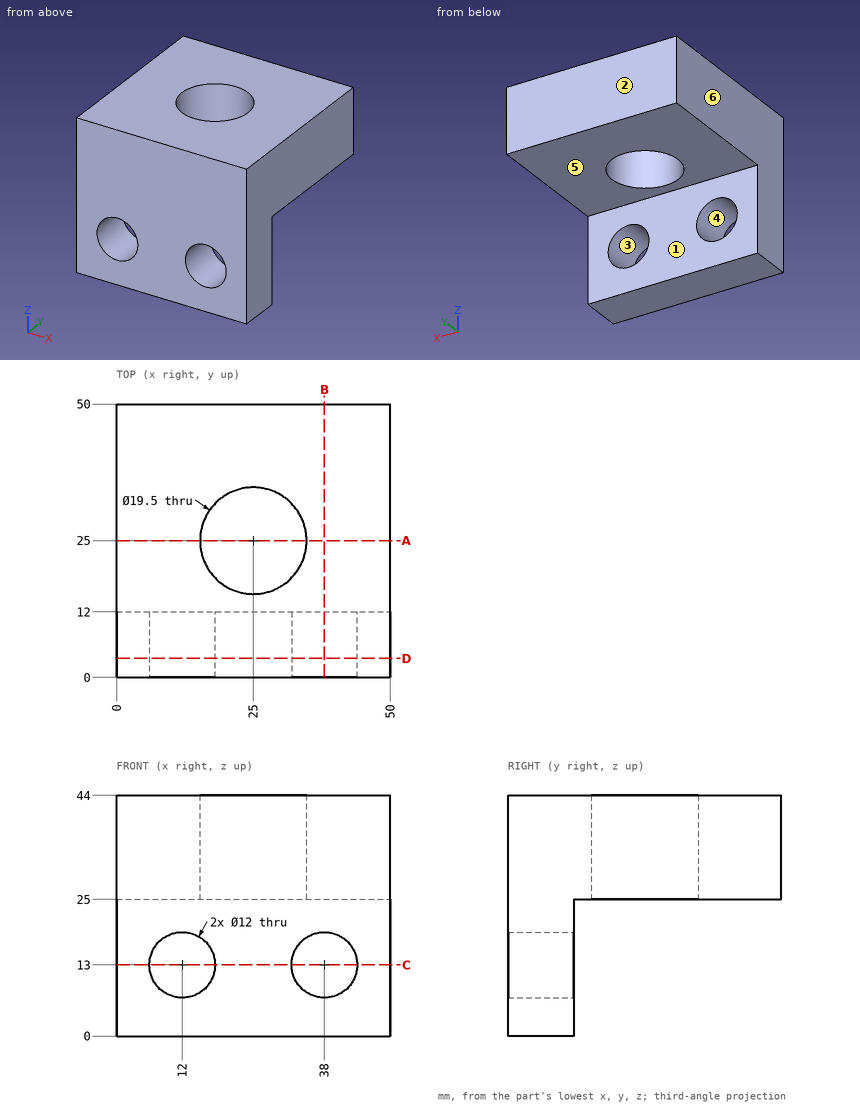
Input: dimensioned drawing with shaded views. Units: mm. Origin: part minimum x, y, z. A direction names the side the tool comes from. Give positions to 0.01 mm unless a question says otherwise; leave off trailing zeros. Write each loop counter-clockwise with the first axis right and the second up, starting at its lowest first coordinate (ties: lowest second). Pieces come first, ordered by that corner, then holes.
1. Material intervals for line 1 along Z through (x, y) = (38, 7); line 2 along Y through (x, z) = (25, 30.5); line 3 along Y through (x, z) = (46.5, 13.5), sorted ascending.
2. First-contact query: pin 1 (3 mm diameter, centred on x = 11, y = 44.5, fed in from -Z); pin 2 (6 mm diameter, centred on x = 30.5, z = 18.5, fed in from +Y). Flat tips, straight axial feed; report the tip coordinate or a pass-through.
3. Pull-direction query (X, two-part tool) for the marked faces 3, 4, 5 and 6; classes: +X half, -X half, draft (parallel to the pull), parting line (faces both ways), or undercut.
4. Access query for the marked faces 1 and 2. Directions: +Z, -Z, +X, -X, +Y, -Y. A direction counts if a zero-diameter tool reaches every point of the face in a straight line with its end or side. Return the directions, or none.
5. Section query D-D (y = 3.5). Return the cut outline in (x, z), then the cut area to 3 significant figures.
6. Section query A-A (y = 25). Return the cut outline in (x, z), then the cut area to 4 significant figures.
7. Section query B-B (x = 38). Return the cut outline in (y, z), then the cut area to 3 significant figures.
8. Section query C-C (z = 13). Return the cut outline in (x, y), then the cut area to 3 significant figures.
Output values:
1. line 1: z = 0 to 7, 19 to 44
1. line 2: y = 0 to 15.25, 34.75 to 50
1. line 3: y = 0 to 12
2. pin 1: stops at z = 25
2. pin 2: stops at y = 12
3. face 3: undercut
3. face 4: undercut
3. face 5: draft
3. face 6: -X half
4. face 1: -Z, +X, -X, +Y
4. face 2: +Z, -Z, +X, -X, +Y
5. outline: (0, 0) - (50, 0) - (50, 44) - (0, 44) - close; hole circle Ø12 at (12, 13); hole circle Ø12 at (38, 13)
5. area: 1,970 mm2
6. outline: (0, 25) - (15.25, 25) - (15.25, 44) - (0, 44) - close; (34.75, 25) - (50, 25) - (50, 44) - (34.75, 44) - close
6. area: 579.5 mm2
7. outline: (0, 0) - (12, 0) - (12, 7) - (0, 7) - close; (0, 19) - (12, 19) - (12, 25) - (50, 25) - (50, 44) - (0, 44) - close
7. area: 1,110 mm2
8. outline: (0, 0) - (6, 0) - (6, 12) - (0, 12) - close; (18, 0) - (32, 0) - (32, 12) - (18, 12) - close; (44, 0) - (50, 0) - (50, 12) - (44, 12) - close
8. area: 312 mm2
